from build123d import *

# Parameters (mm, degrees)
SALIENTE_EXTRUIR1_DEPTH = 20
CROQUIS2_W              = 10
CROQUIS2_H              = 3.08
CROQUIS2_W_2            = 3.08
CROQUIS2_H_2            = 10
CORTAR_EXTRUIR2_DEPTH   = 20


with BuildPart() as part:
    # Croquis1 → Saliente-Extruir1 (new body)
    with BuildSketch(Plane(origin=(0, 0, 0), x_dir=(1, 0, 0), z_dir=(0, 1, 0))):
        Polygon((7.5, 12.5), (7.5, 7.5), (12.5, 7.5), (12.5, -12.5), (-12.5, -12.5), (-12.5, 12.5), align=None)
    extrude(amount=SALIENTE_EXTRUIR1_DEPTH)

    # Croquis2 → Cortar-Extruir2 (cut)
    with BuildSketch(Plane(origin=(0, 20, 0), x_dir=(1, 0, 0), z_dir=(0, 1, 0))):
        with Locations((7.5, -7.96)):
            Rectangle(CROQUIS2_W, CROQUIS2_H)
        with Locations((-7.96, 7.5)):
            Rectangle(CROQUIS2_W_2, CROQUIS2_H_2)
    extrude(amount=-CORTAR_EXTRUIR2_DEPTH, mode=Mode.SUBTRACT)


solid = part.part
Geometry check sheet. Reference: the model listing, model coordinates, mm. A direction names the side the tool comes from. Round coordinates to 2 decimals unless told otherwise and drop trailing zeros. Order: outer loops, then holes, each group sorted by start corner. A loop starts at its lowest first (then second) coordinate and runs counter-clockwise, first axis right, second up. Notation, with made-up numbers: M 6.25,39.25 L 53.25,39.25 A20 cw 53.25,74.25 Z; hole C 65,33.5 d9. An arc over 180 degrees is marked long. Answer in a Markdown table with one row per item.
(1) Sectioned sample at B-B, the plane x = 10.5. Record the cut outline in (y, z).
Responses:
| item | result |
|---|---|
| outline | M 0,-7.5 L 20,-7.5 L 20,6.42 L 0,6.42 Z; M 0,9.5 L 20,9.5 L 20,12.5 L 0,12.5 Z |
(2) Go/stop test with flat-tipped pins: P1, Ø3, axis at y = 13.5, z = -10, coming from the +X side; P2, Ø0.9, axis at y = 10.5, z = 8, coming from the +X side; P3, Ø1.5, axis at x = 9, y = 13.5, coming from the -Z side. Record where each tip stops, or that it passes through.
Responses:
| item | result |
|---|---|
| P1 | stops at x = 7.5 |
| P2 | stops at x = 2.5 |
| P3 | stops at z = -7.5 |
(3) Sectioned sample at C-C, the plane y = 7.25. Record the cut outline in (x, z).
Responses:
| item | result |
|---|---|
| outline | M -12.5,-12.5 L -9.5,-12.5 L -9.5,-2.5 L -6.42,-2.5 L -6.42,-12.5 L 7.5,-12.5 L 7.5,-7.5 L 12.5,-7.5 L 12.5,6.42 L 2.5,6.42 L 2.5,9.5 L 12.5,9.5 L 12.5,12.5 L -12.5,12.5 Z |
(4) Draft check along Z on faces 4 (the face through (7, 10, 6.42)), 5 (the face through (10, 10, -7.5)), 6 (the face through (7, 10, 9.5)), 7 (the face through (12.5, 10, 11)). Enter one of: released by +Z, released by -Z, zero draft, split by the parting line, or undercut.
Responses:
| item | result |
|---|---|
| face 4 | undercut |
| face 5 | released by -Z |
| face 6 | undercut |
| face 7 | zero draft |
(5) Sectioned sample at A-A, the plane z = -5.25. Record the cut outline in (x, y), and give its area (3 significant figures).
Responses:
| item | result |
|---|---|
| outline | M -12.5,0 L -9.5,0 L -9.5,20 L -12.5,20 Z; M -6.42,0 L 12.5,0 L 12.5,20 L -6.42,20 Z |
| area | 438 mm² |
(6) Sectioned sample at D-D, the plane x = -7. Record the cut outline in (y, z).
Responses:
| item | result |
|---|---|
| outline | M 0,-2.5 L 20,-2.5 L 20,12.5 L 0,12.5 Z |
(7) Tool access check on faces 1 (the face through (-6.42, 10, -7)), 2 (the face through (7.5, 10, -10)), 3 (the face through (2.5, 10, 8)). Record the directions out of +Z, -Z, +X, -X, +Y, -Y that give a thin tool (end or side, any length) a straight path to the whole face; none if there is none.
Responses:
| item | result |
|---|---|
| face 1 | -Z, +Y, -Y |
| face 2 | -Z, +X, +Y, -Y |
| face 3 | +X, +Y, -Y |
(8) Scan lines: probe 1 along X at (y, z) = (2, -5.5); probe 2 along Z at (x, y) = (4.5, 8); probe 3 along X at (y, z) = (15.25, -8.5). Record each from-to range of solid material in increasing order. Write a range as from..to.
Responses:
| item | result |
|---|---|
| probe 1 | x = -12.5..-9.5, -6.42..12.5 |
| probe 2 | z = -12.5..6.42, 9.5..12.5 |
| probe 3 | x = -12.5..-9.5, -6.42..7.5 |
